from build123d import *

# Parameters (mm, degrees)
SKETCH_1_R      = 1.5
EXTRUDE_1_DEPTH = 2.4
SKETCH_4_R      = 2.4
SKETCH_4_R_2    = 1.5
EXTRUDE_3_DEPTH = 1.2
FILLET_5_R      = 0.3
SCALE_1_SCALE   = 2


with BuildPart() as part:
    # 草图1 → 凸台-拉伸1 (new body)
    with BuildSketch(Plane(origin=(0, 0, 0), x_dir=(1, 0, 0), z_dir=(0, 1, 0))):
        Polygon((0, 3.175426481), (-2.75, 1.58771324), (-2.75, -1.58771324), (0, -3.175426481), (2.75, -1.58771324), (2.75, 1.58771324), align=None)
        with Locations(Location((0, 0, 0), (0, 0, 270))):
            Circle(SKETCH_1_R, mode=Mode.SUBTRACT)
    extrude(amount=EXTRUDE_1_DEPTH)

    # 草图3 → 切除-旋转7 (revolve, cut)
    with BuildSketch(Plane(origin=(0, 0, 0), x_dir=(0, 0, -1), z_dir=(1, 0, 0))):
        Polygon((0.384303775, 7.2), (4.083483307, 7.2), (4.083483307, -4.8), (0.297701235, -4.8), (0.297701235, -4.284366336), (3.464101615, 1.2), (0.384303775, 6.534366336), align=None)
    revolve(axis=Axis((0, 2.4, 0), (0, -1, 0)), mode=Mode.SUBTRACT)

    # 草图4 → 凸台-拉伸3 (add)
    with BuildSketch(Plane(origin=(0, 2.4, 0), x_dir=(1, 0, 0), z_dir=(0, 1, 0))):
        with Locations(Location((0, 0, 0), (0, 0, 270))):
            Circle(SKETCH_4_R)
        with Locations(Location((0, 0, 0), (0, 0, 270))):
            Circle(SKETCH_4_R_2, mode=Mode.SUBTRACT)
    extrude(amount=EXTRUDE_3_DEPTH)

    # 圆角5
    fillet_5_edges = [part.edges().sort_by_distance(p)[0] for p in [
        (0, 3.6, -2.4),
    ]]
    fillet(fillet_5_edges, radius=FILLET_5_R)


with BuildPart() as part_1:
    # 缩放比例1: scaled about (0, 1.599672866, 1e-09)
    add(part.part.scale(SCALE_1_SCALE).moved(Location((0, -1.599672866, -1e-09))))


solid = part_1.part
Verification items for the finished model (mm, model axes). A direction names the side the tool comes from. Round coordinates to 2 decimals unless told otherwise and drop trailing zeros. Order: outer loops, then holes, each group sorted by start corner. A loop starts at its lowest first (then second) coordinate and runs counter-clockwise, first axis right, second up.
1. Thickness scan on L1, parallel to X at y = 0, z = 0; L2, parallel to X at y = 3.25, z = 0; L3, parallel to Y at x = -4.25, z = 0.25. Record the ranges inside material, lowest first.
Final values:
L1: x = -5.5 to -3, 3 to 5.5
L2: x = -4.8 to -3, 3 to 4.8
L3: y = -1.6 to 5.6
2. Release check for a two-part mould opening along Z. For faces 3 (the cylindrical face through (-1.8, 1.9, -2.4)), 4 (the conical face through (-4.973, 2.821, 2.909)), 5 (the conical face through (-5.01, 2.82, -2.85)) record: +Z half, -Z half, draft (parallel to the pull), parting line (faces both ways), or undercut.
Final values:
face 3: undercut
face 4: +Z half
face 5: -Z half
3. Access from +Z, -Z, +X, -X, +Y, -Y to the whole of each face (thin tool, end or side, straight path). Record for faces 1 (the flat face through (0, 3.2, 5)), 2 (the conical face through (5.015, -1.201, 2.858)).
Final values:
face 1: +Y
face 2: +Z, +X, -Y
4. Go/stop test with flat-tipped pins: P1, Ø1.5, axis at x = -4, z = -4, coming from the +Y side; P2, Ø3, axis at x = 4, y = -1, coming from the -Z side; P3, Ø1.5, axis at x = -0.5, z = -2.5, coming from the -Y side. Record where each tip stops, or that it passes through.
Final values:
P1: stops at y = 3.2
P2: stops at z = -4.91
P3: stops at y = -1.6
5. Section check A-A on y = 1. Record the cut outline in (x, z).
Final values:
outline: (-5.5, -3.18) - (0, -6.35) - (5.5, -3.18) - (5.5, 3.18) - (0, 6.35) - (-5.5, 3.18) - close; hole circle Ø6 at (0, 0)
